Work out the finished part from the listing and answer in its coordinate system (mm). Round coordinates to 2 decimals unless told otherwise and drop trailing zeros. Write each loop counter-clockwise with the first axis right and the second up, starting at its lowest first coordinate (ties: lowest second). Pieces come first, ordered by that corner, then holes. Notation, with made-up numbers: (82.5, 16) - (105.5, 16) arc R31 cw to (105.5, 50) - close; hole circle Ø3 at (68.25, 77.5). An arc over 180 degrees is marked (long way). Answer as a JSON object with one key per item and string values.
```python
from build123d import *

# Parameters (mm, degrees)
BOSS_EXTRUDE1_DEPTH = 12
SKETCH2_R           = 5.795
CUT_EXTRUDE1_DEPTH  = 10


with BuildPart() as part:
    # Sketch1 → Boss-Extrude1 (new body)
    with BuildSketch(Plane.XY):
        with BuildLine():
            Line((-125, 130), (125, 130))
            ThreePointArc((125, 130), (128.535533906, 128.535533906), (130, 125))
            Line((130, 125), (130, -125))
            ThreePointArc((130, -125), (128.535533906, -128.535533906), (125, -130))
            Line((125, -130), (-125, -130))
            ThreePointArc((-125, -130), (-128.535533906, -128.535533906), (-130, -125))
            Line((-130, -125), (-130, 125))
            ThreePointArc((-130, 125), (-128.535533906, 128.535533906), (-125, 130))
        make_face()
    extrude(amount=BOSS_EXTRUDE1_DEPTH)

    # Sketch2 → Cut-Extrude1 (cut)
    with BuildSketch(Plane.XY.offset(12)):
        Circle(SKETCH2_R)
    extrude(amount=-CUT_EXTRUDE1_DEPTH, mode=Mode.SUBTRACT)


solid = part.part
```
Item 1: Consider line 1 along Y through (x, z) = (2, 5.75). Determine where the line is inside the solid, lowest interval first.
Results found:
{"line 1": "-130 to -5.44, 5.44 to 130"}
Item 2: Determine the mould class of faces 1 (the flat face through (2, 2, 0)), 2 (the flat face through (-2, 130, 6)), 3 (the flat face through (0, 0, 2)), 4 (the cylindrical face through (5.527, 1.741, 7.07)) for opening direction Y: pulls with the +Y half, pulls with the -Y half, needs draft (parallel to the pull), parting line crosses it, or undercut.
Results found:
{"face 1": "needs draft", "face 2": "pulls with the +Y half", "face 3": "undercut", "face 4": "undercut"}
Item 3: A cutting plane is placed at A-A (x = 0). Write down the section's boundary in (y, z) (3 decimals), and give its area (3 significant figures).
Results found:
{"outline": "(-130, 0) - (130, 0) - (130, 12) - (5.795, 12) - (5.795, 2) - (-5.795, 2) - (-5.795, 12) - (-130, 12) - close", "area": "3,000 mm²"}
